Here's the drawing with two shaded views (mm, measured from the low corner). I have some questions. A direction names the side the tool comes from. Coordinates: 2 decimals unless noted, no trailing zeros. Loops run counter-clockwise (first coordinate to the right, second up) from the corner with the lowest first, then second, coordinate; pieces in that order, holes last. Notation, with made-up numbers: (27, 84) - (43, 84) arc R17 ccw to (43, 107) - close; hole circle Ø4 at (62, 56). An arc over 180 degrees is marked (long way). Use a Markdown table: item, result.
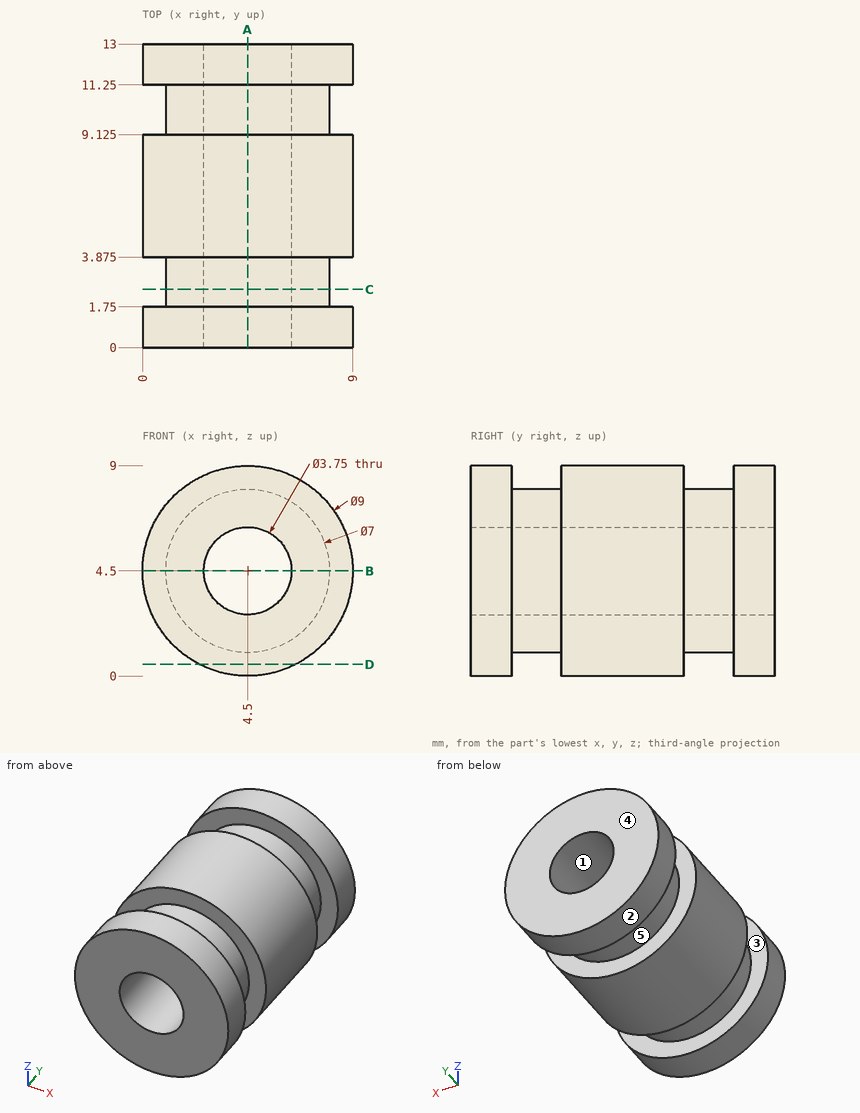
Q1. I want a section at C-C, the plane y = 2.5. Write out the boundary of the cut face in (x, z) (3 decimals), then the cut area to 3 significant figures.
Check values:
| item | result |
|---|---|
| outline | circle Ø7 at (4.5, 4.5); hole circle Ø3.75 at (4.5, 4.5) |
| area | 27.4 mm^2 |
Q2. I want a section at A-A, the plane x = 4.5. Write out the boundary of the cut face in (y, z) (3 decimals), then the cut area to 4 significant figures.
Check values:
| item | result |
|---|---|
| outline | (0, 0) - (1.75, 0) - (1.75, 1) - (3.875, 1) - (3.875, 0) - (9.125, 0) - (9.125, 1) - (11.25, 1) - (11.25, 0) - (13, 0) - (13, 2.625) - (0, 2.625) - close; (0, 6.375) - (13, 6.375) - (13, 9) - (11.25, 9) - (11.25, 8) - (9.125, 8) - (9.125, 9) - (3.875, 9) - (3.875, 8) - (1.75, 8) - (1.75, 9) - (0, 9) - close |
| area | 59.75 mm^2 |
Q3. Will these pins go through, and if not, where does the flat tip stop? P1, Ø5, axis at x = 7, y = 3, coming from the -Z side; P2, Ø3.5, axis at x = 4.5, z = 4.5, coming from the +Y side; P3, Ø3, axis at y = 9, z = 6.5, coming from the +X side; P4, Ø2, axis at x = 7.5, y = 8.5, coming from the -Z side.
Check values:
| item | result |
|---|---|
| P1 | z = 0 |
| P2 | through |
| P3 | x = 8.97 |
| P4 | z = 0.47 |
Q4. I want a section at B-B, the plane z = 4.5. Write out the boundary of the cut face in (x, y) (3 decimals).
Check values:
| item | result |
|---|---|
| outline | (0, 0) - (2.625, 0) - (2.625, 13) - (0, 13) - (0, 11.25) - (1, 11.25) - (1, 9.125) - (0, 9.125) - (0, 3.875) - (1, 3.875) - (1, 1.75) - (0, 1.75) - close; (6.375, 0) - (9, 0) - (9, 1.75) - (8, 1.75) - (8, 3.875) - (9, 3.875) - (9, 9.125) - (8, 9.125) - (8, 11.25) - (9, 11.25) - (9, 13) - (6.375, 13) - close |
Q5. I want a section at D-D, the plane z = 0.5. Write out the boundary of the cut face in (x, y) (3 decimals).
Check values:
| item | result |
|---|---|
| outline | (2.438, 0) - (6.562, 0) - (6.562, 1.75) - (2.438, 1.75) - close; (2.438, 3.875) - (6.562, 3.875) - (6.562, 9.125) - (2.438, 9.125) - close; (2.438, 11.25) - (6.562, 11.25) - (6.562, 13) - (2.438, 13) - close |
Q6. If we mould it in two halves opening along Z, with no side actions, what happens to the marked faces 1, 2 and 3? For each: pulls with the +Z half, pulls with the -Z half, needs draft (parallel to the pull), parting line crosses it, or undercut.
Check values:
| item | result |
|---|---|
| face 1 | undercut |
| face 2 | parting line crosses it |
| face 3 | needs draft |
Q7. Please list where these lines run through material, in increasing order: L1, parallel to Y at x = 4.25, z = 0.5 (3 decimals); L2, parallel to Z at x = 4.5, y = 4.75 (3 decimals); L3, parallel to X at y = 3.5, z = 4.5 (3 decimals). Write a range as from..to.
Check values:
| item | result |
|---|---|
| L1 | 0..1.75, 3.875..9.125, 11.25..13 |
| L2 | 0..2.625, 6.375..9 |
| L3 | 1..2.625, 6.375..8 |
Q8. Which directions (+Z, -Z, +X, -X, +Y, -Y) give clear straight access to the entire face, cutting with the end or side of a thin tool? Please do the marked faces 4 and 5.
Check values:
| item | result |
|---|---|
| face 4 | +Z, -Z, +X, -X, +Y |
| face 5 | none |
